Source: three-view drawing plus pictorial views. Frame: mm from the lowest corner of the part. Give positions to 0.01 mm unless a question says otherwise; leave off trailing zeros. Order: outer loops, then holes, each group sorted by start corner. A loop starts at its lowest first (then second) coordinate and runs counter-clockwise, first axis right, second up. Notation, with made-up numbers: (40.5, 80) - (55.5, 80) arc R19 cw to (55.5, 112) - close; hole circle Ø5 at (16, 44.25). An arc over 180 degrees is marked (long way). Answer in a Markdown table with one row per item. Add a question column.
1. Mould query, pull axis X, two halves, no side actions, for the marked faces 1, 2, 3 and 4. Classes: released by +X, released by -X, zero draft, split by the parting line, or undercut.
2. Section query D-D on z = 9. Return loops of the section in (x, y).
3. Section query A-A on y = 21. Return loops of the section in (x, z).
4. Section query C-C on z = 2.75. Return loops of the section in (x, y).
5. Section query B-B on x = 21. Return loops of the section in (y, z), and give its area (3 significant figures).
6. Contact query for flat-ended pins moving along their axis: pin 1 (6 mm diameter, centred on x = 6, z = 14.5, fed in from +Y); pin 2 (1 mm diameter, centred on y = 10, z = 9, fed in from +X); pin 3 (3.5 mm diameter, centred on x = 21, z = 9, fed in from +Y); pin 4 (17.5 mm diameter, centred on x = 21, y = 21, fed in from +Z). Output: stop coordinate, or through.
7. Ray query, line 1 (Y direction, x = 21, z = 14.25); line 2 (Z direction, x = 21, y = 5.5); line 3 (Y direction, x = 15, z = 3.5). Return the intervals inside material, ascending. Write a range as [from, to].
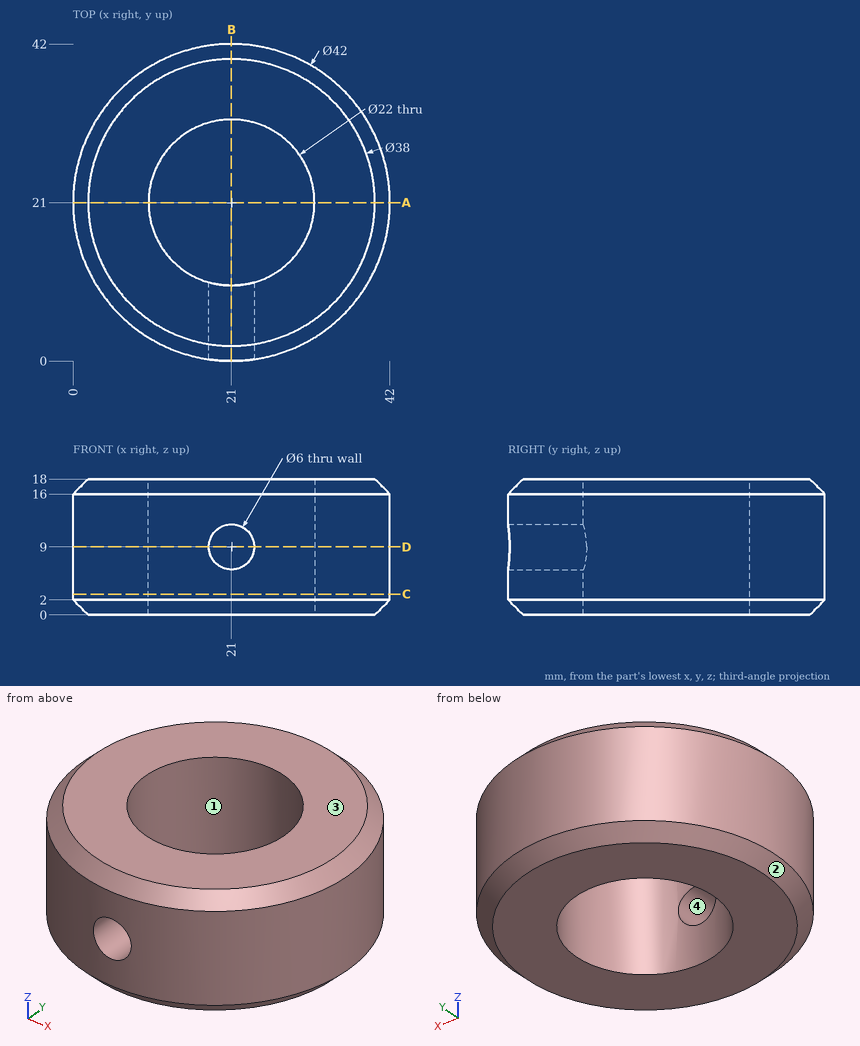
Answer:
| question | item | result |
|---|---|---|
| 1 | face 1 | undercut |
| 1 | face 2 | split by the parting line |
| 1 | face 3 | zero draft |
| 1 | face 4 | undercut |
| 2 | outline | (18, 0.22) - (18, 10.42) arc R11 cw (long way) to (24, 10.42) - (24, 0.22) arc R21 ccw (long way) to start |
| 3 | outline | (0, 2) - (2, 0) - (10, 0) - (10, 18) - (2, 18) - (0, 16) - close; (32, 0) - (40, 0) - (42, 2) - (42, 16) - (40, 18) - (32, 18) - close |
| 4 | outline | circle Ø42 at (21, 21); hole circle Ø22 at (21, 21) |
| 5 | outline | (0, 2) - (2, 0) - (10, 0) - (10, 6) - (0, 6) - close; (0, 12) - (10, 12) - (10, 18) - (2, 18) - (0, 16) - close; (32, 0) - (40, 0) - (42, 2) - (42, 16) - (40, 18) - (32, 18) - close |
| 5 | area | 292 mm² |
| 6 | pin 1 | stops at y = 38.23 |
| 6 | pin 2 | stops at x = 39.19 |
| 6 | pin 3 | stops at y = 42 |
| 6 | pin 4 | passes through |
| 7 | line 1 | y = [0, 10], [32, 42] |
| 7 | line 2 | z = [0, 6], [12, 18] |
| 7 | line 3 | y = [0.88, 11.78], [30.22, 41.12] |
